The model under review builds one solid part; all positions refer to its coordinate system, in mm. A direction names the side the tool comes from. Give positions to 0.01 mm unless a question says otherwise; leave off trailing zeros. Loops run counter-clockwise (first coordinate to the right, second up) from the corner with the lowest first, then second, coordinate; pieces in that order, holes last. Notation, with made-up numbers: (-9.5, -26) - (-2.5, -26) arc R6 ccw to (-2.5, -21) - close; hole circle Ø5 at (86, 30). An arc over 180 degrees is marked (long way). Answer as a JSON object with one key per item and string values.
from build123d import *

# Parameters (mm, degrees)
EXTRUDE1_DEPTH                                 = 5
SKETCH2_R                                      = 10
EXTRUDE2_DEPTH                                 = 10
BROCA_DE_ROSQUEAR_PARA_TARRAXA_DE_M2_2X0_D     = 1.75
BROCA_DE_ROSQUEAR_PARA_TARRAXA_DE_M2_2X0_DEPTH = 5
BROCA_DE_ROSQUEAR_PARA_TARRAXA_DE_M2_2X0_TIP   = 0.525753042


with BuildPart() as part:
    # Sketch1 → Extrude1 (new body, symmetric)
    with BuildSketch(Plane.XY):
        with BuildLine():
            Line((11.498532289, 11.006151708), (-15.451429048, -27.482381858))
            ThreePointArc((-15.451429048, -27.482381858), (-29.378713855, -29.938137938), (-31.834469934, -16.010853131))
            Line((-31.834469934, -16.010853131), (-4.884508596, 22.477680435))
            ThreePointArc((-4.884508596, 22.477680435), (4.05057718, 30.313540355), (15.594292511, 33.138269526))
            Line((15.594292511, 33.138269526), (61.357050509, 33.138269526))
            Line((61.357050509, 33.138269526), (61.357050509, 13.138269526))
            Line((61.357050509, 13.138269526), (15.594292511, 13.138269526))
            ThreePointArc((15.594292511, 13.138269526), (13.285549445, 12.573323692), (11.498532289, 11.006151708))
        make_face()
        with BuildLine():
            Line((-26.919557668, -19.45231175), (-6.844382396, 9.218009801))
            ThreePointArc((-6.844382396, 9.218009801), (-1.273468473, 10.200312232), (-0.291166042, 4.62939831))
            Line((-0.291166042, 4.62939831), (-20.366341314, -24.04092324))
            ThreePointArc((-20.366341314, -24.04092324), (-25.937255237, -25.023225672), (-26.919557668, -19.45231175))
        make_face(mode=Mode.SUBTRACT)
    extrude(amount=EXTRUDE1_DEPTH, both=True)

    # Sketch2 → Extrude2 (add)
    with BuildSketch(Plane(origin=(0, 33.138269526, 0), x_dir=(1, 0, 0), z_dir=(0, 1, 0))):
        with BuildLine():
            Line((61.357050509, 5), (15.594292511, 5))
            Line((15.594292511, 5), (15.594292511, -5))
            Line((15.594292511, -5), (26.357050509, -5))
            ThreePointArc((26.357050509, -5), (35.195885274, -8.661165235), (38.857050509, -17.5))
            ThreePointArc((38.857050509, -17.5), (77.266953086, -33.409902577), (61.357050509, 5))
        make_face()
        with Locations(Location((61.357050509, -17.5, 0), (0, 0, 180))):  # turned: the seam where the file's is
            Circle(SKETCH2_R, mode=Mode.SUBTRACT)
    extrude(amount=-EXTRUDE2_DEPTH)

    # Broca de rosquear para tarraxa de M2.2x0.451
    with Locations(Plane(origin=(61.357050509, 18.138269526, 0), x_dir=(0, 1, 0), z_dir=(1, 0, 0))):
        with Locations((0, 0)):
            Hole(BROCA_DE_ROSQUEAR_PARA_TARRAXA_DE_M2_2X0_D / 2, depth=BROCA_DE_ROSQUEAR_PARA_TARRAXA_DE_M2_2X0_DEPTH)
            with Locations((0, 0, -(BROCA_DE_ROSQUEAR_PARA_TARRAXA_DE_M2_2X0_DEPTH + BROCA_DE_ROSQUEAR_PARA_TARRAXA_DE_M2_2X0_TIP / 2))):  # 118° drill point
                Cone(0, BROCA_DE_ROSQUEAR_PARA_TARRAXA_DE_M2_2X0_D / 2, BROCA_DE_ROSQUEAR_PARA_TARRAXA_DE_M2_2X0_TIP, mode=Mode.SUBTRACT)


solid = part.part
Q1. Consider section B-B, the plane z = 22.5. State the section outline as (x, y) points.
Results:
{"outline": "(39.42, 23.14) - (52.7, 23.14) - (52.7, 33.14) - (39.42, 33.14) - close; (70.02, 23.14) - (83.29, 23.14) - (83.29, 33.14) - (70.02, 33.14) - close"}
Q2. Clearance check with flat-ended pins moving along their axes: pin 1 Ø23 at (x, z) = (61.36, 17.5) entering from +Y; pin 2 Ø3 at (y, z) = (16.5, 2) entering from +X; pin 3 Ø8 at (y, z) = (-6, 4.5) entering from +X; pin 4 Ø8 at (y, z) = (-24, 1.5) entering from +X. State where each tip first meets the part, or that it passes through.
Results:
{"pin 1": "stops at y = 33.14", "pin 2": "stops at x = 61.36", "pin 3": "stops at x = 2.39", "pin 4": "stops at x = -10.21"}
Q3. Consider section C-C, the plane x = -12.5. State the section outline as (y, z) points, plus the area to 3 significant figures.
Results:
{"outline": "(-23.27, -5) - (-12.81, -5) - (-12.81, 5) - (-23.27, 5) - close; (1.14, -5) - (11.6, -5) - (11.6, 5) - (1.14, 5) - close", "area": "209 mm^2"}
Q4. Consider section D-D, the plane z = 30.5. State the section outline as (x, y) points, plus the area to 3 significant figures.
Results:
{"outline": "(42.99, 23.14) - (79.72, 23.14) - (79.72, 33.14) - (42.99, 33.14) - close", "area": "367 mm^2"}
Q5. For faces 1 (the face through (14, 15, -5)), 2 (the face through (61.357, 17, 0)), 3 (the face through (-10.19, -9.51, 0.07)), list the 3-axis set-ups (+Z, -Z, +X, -X, +Y, -Y) from which the entire face can be reached by the end or side of a thin tool; tool diameter is ignored.
Results:
{"face 1": "-Z, +X, -X, +Y, -Y", "face 2": "+Z, -Z, +X, -Y", "face 3": "+Z, -Z"}
Q6. To check wall thickness, follow probe 1 along Y at (x, z) = (57.85, 0); probe 2 along X at (y, z) = (28, 17); probe 3 along Z at (x, y) = (-11.5, -14). State the ranges of each line that lie inside material, in increasing order. Write a range as [from, to].
Results:
{"probe 1": "y = [13.14, 17.26], [19.01, 33.14]", "probe 2": "x = [38.85, 51.37], [71.34, 83.85]", "probe 3": "z = [-5, 5]"}
Q7. Consider section A-A, the plane x = 60. State how many separate pieces and enclosed holes the cut face has, plus the area to 3 significant figures.
Results:
{"separate pieces": "2", "enclosed holes": "1", "area": "349 mm^2"}
Q8. The part is to be moulded in two halves that separate along X. For faces 4 (the face through (7, 8, 5)), 5 (the face through (3.902, 30.235, 0.07)), 6 (the face through (-25.865, -25.073, 0.07)), say which applies: +X half, -X half, draft (parallel to the pull), parting line (faces both ways), or undercut.
Results:
{"face 4": "draft", "face 5": "-X half", "face 6": "undercut"}
